from build123d import *

# Parameters (mm, degrees)
F0_R     = 14
F1_DEPTH = 2
F2_DEPTH = 40
F3_SIZE  = 2


with BuildPart() as f1:
    # F0 (on Top) → F1 (new body)
    with BuildSketch(Plane.XY):
        Polygon((12.351223, -17), (19.984699, 6.493422), (0, 21.013156), (-19.984699, 6.493422), (-12.351223, -17), align=None)
        Circle(F0_R, mode=Mode.SUBTRACT)
        Circle(F0_R)
    extrude(amount=F1_DEPTH)

    # F0 (on Top) → F2 (join)
    with BuildSketch(Plane.XY):
        Polygon((12.351223, -17), (19.984699, 6.493422), (0, 21.013156), (-19.984699, 6.493422), (-12.351223, -17), align=None)
        Circle(F0_R, mode=Mode.SUBTRACT)
    extrude(amount=F2_DEPTH)

    # F3
    f3_edges = [f1.edges().sort_by_distance(p)[0] for p in [
        (16.167961, -5.253289, 40),
        (9.992349, 13.753289, 40),
        (-9.992349, 13.753289, 40),
        (-16.167961, -5.253289, 40),
        (0, -17, 40),
        (16.167961, -5.253289, 0),
        (9.992349, 13.753289, 0),
        (-16.167961, -5.253289, 0),
        (0, -17, 0),
        (-9.992349, 13.753289, 0),
    ]]
    chamfer(f3_edges, length=F3_SIZE)


solid = f1.part
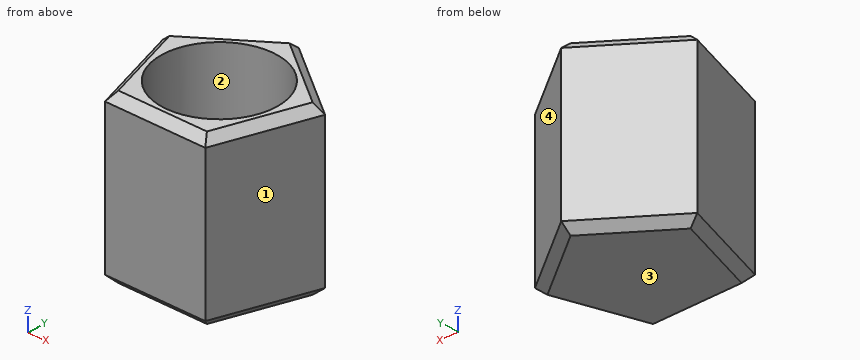
Geometry: final body of the model. Coordinates: model frame, mm. Face numbers are marked on the shaded views. Round coordinates to 2 decimals unless told otherwise and drop trailing zeros. Order: outer loops, then holes, each group sorted by start corner. A loop starts at its lowest first (then second) coordinate and runs counter-clockwise, first axis right, second up.
Q1. Section A-A, the plane z = 18.5. Output: boundary loops of the cut face in (x, y).
Result sheet:
outline: (-19.98, 6.49) - (-12.35, -17) - (12.35, -17) - (19.98, 6.49) - (0, 21.01) - close; hole circle Ø28 at (0, 0)
Q2. Pin query (flat end, axial travel): pin 1 (6 mm diameter, centred on y = 12, z = 5, fed in from +X); pin 2 (6 mm diameter, centred on x = -3.5, z = 13.5, fed in from +Y); pin 3 (8.5 mm diameter, centred on x = -0.5, y = 1, fed in from +Z). Return the tip coordinate at first contact, or that it passes through.
Result sheet:
pin 1: stops at x = 16.53
pin 2: stops at y = 20.65
pin 3: stops at z = 2
Q3. Mould query, pull axis Y, two halves, no side actions, for the marked faces 1, 2, 3 and 4. Classes: released by +Y, released by -Y, zero draft, split by the parting line, or undercut.
Result sheet:
face 1: released by -Y
face 2: undercut
face 3: zero draft
face 4: released by +Y
Q4. Section D-D, the plane x = 15. Output: boundary loops of the cut face in (y, z), and give its area (3 significant figures).
Result sheet:
outline: (-8.85, 2) - (-2.38, 0) - (7.64, 0) - (10.12, 2) - (10.12, 38) - (7.64, 40) - (-2.38, 40) - (-8.85, 38) - close
area: 741 mm2
Q5. Section C-C, the plane y = 12. Output: boundary loops of the cut face in (x, z), and give its area (3 significant figures).
Result sheet:
outline: (-12.41, 2) - (-9, 0) - (9, 0) - (12.41, 2) - (12.41, 38) - (9, 40) - (7.21, 40) - (7.21, 2) - (-7.21, 2) - (-7.21, 40) - (-9, 40) - (-12.41, 38) - close
area: 431 mm2
Q6. Section B-B, the plane x = 7. Output: boundary loops of the cut face in (y, z).
Result sheet:
outline: (-17, 2) - (-15, 0) - (13.46, 0) - (15.93, 2) - (15.93, 38) - (13.46, 40) - (12.12, 40) - (12.12, 2) - (-12.12, 2) - (-12.12, 40) - (-15, 40) - (-17, 38) - close
Q7. Material intervals for probe 1 along Y at (x, z) = (0, 17); probe 2 along X at (y, z) = (10.5, 9); probe 3 along Z at (x, y) = (-5.5, 9.5), sorted ascending.
Result sheet:
probe 1: y = -17 to -14, 14 to 21.01
probe 2: x = -14.47 to -9.26, 9.26 to 14.47
probe 3: z = 0 to 2
